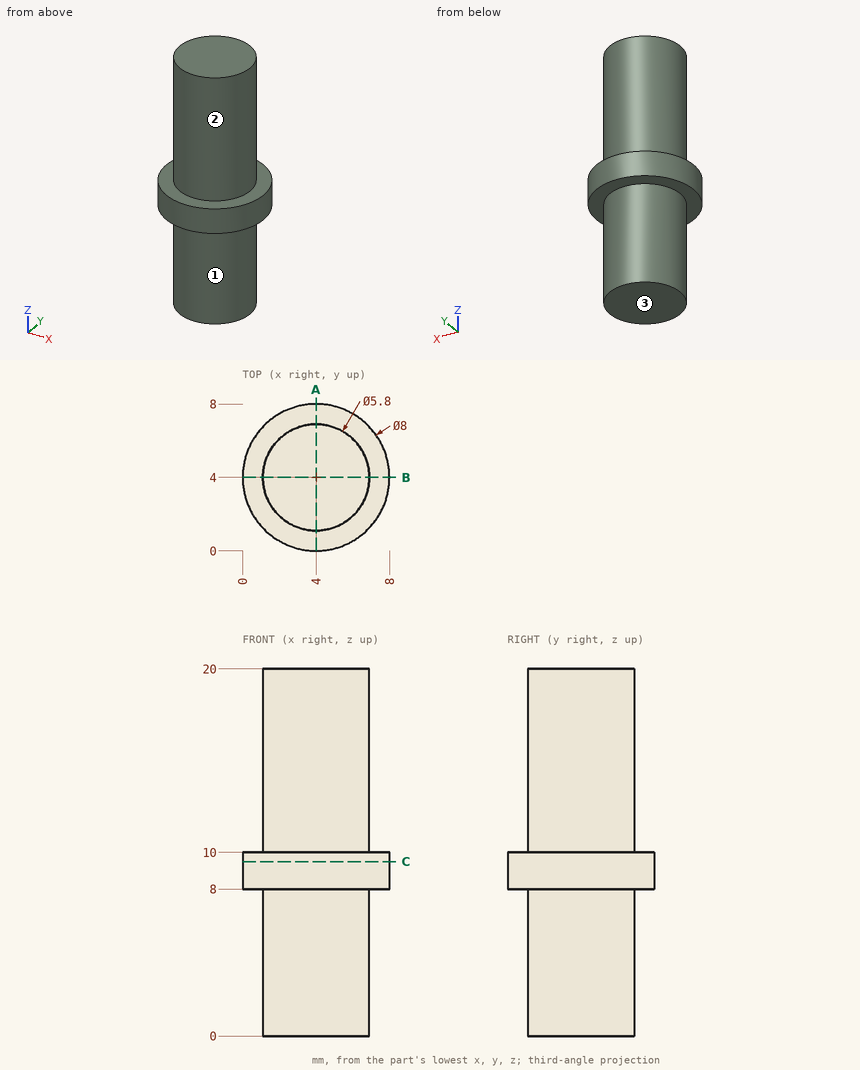
Part print with two shaded views. Sizes in mm from the minimum x, y, z corner. A direction names the side the tool comes from. Coordinates: 2 decimals unless noted, no trailing zeros. Write each loop counter-clockwise with the first axis right and the second up, starting at its lowest first coordinate (ties: lowest second). Pieces come first, ordered by that corner, then holes.
1. Drill centre lines: probe 1 along X at (y, z) = (4, 12.25); probe 2 along Z at (x, y) = (1.5, 1.75); probe 3 along Y at (x, z) = (2.25, 3.5). Where is each one in solid material? Low to high.
Answer block:
probe 1: x = 1.1 to 6.9
probe 2: z = 8 to 10
probe 3: y = 1.69 to 6.31
2. Band-saw the part on A-A, the plane x = 4. Give the cut face in (y, z).
Answer block:
outline: (0, 8) - (1.1, 8) - (1.1, 0) - (6.9, 0) - (6.9, 8) - (8, 8) - (8, 10) - (6.9, 10) - (6.9, 20) - (1.1, 20) - (1.1, 10) - (0, 10) - close
3. Drop a flat-ended pin along its axis: pin 1 (1.5 mm diameter, centred on x = 4, z = 6.5, fed in from -Y). Give the stop position or say it passes through.
Answer block:
pin 1: stops at y = 1.1
4. 3-axis set-ups, long thin cutter, end or side, ignore diameter. For the marked faces 1, 2 and 3: which of +Z, -Z, +X, -X, +Y, -Y reach the whole face in a straight line?
Answer block:
face 1: -Z
face 2: +Z
face 3: -Z, +X, -X, +Y, -Y
5. Band-saw the part on C-C, the plane z = 9.5. Give the cut face in (x, y).
Answer block:
outline: circle Ø8 at (4, 4)
